Check sheet for the modelled part. Datum: model origin and axes. Units: mm. A direction names the side the tool comes from. Give positions to 0.01 mm unless a question says otherwise; leave off trailing zeros. Order: outer loops, then holes, each group sorted by start corner. A loop starts at its lowest first (then second) coordinate and runs counter-clockwise, first axis right, second up.
```python
from build123d import *

# Parameters (mm, degrees)
SKETCH176_R     = 2.25
PAD098_DEPTH    = 4
SKETCH177_W     = 20.5
SKETCH177_H     = 20.5
POCKET040_DEPTH = 2
CHAMFER002_SIZE = 0.8
FILLET008_R     = 1.5


with BuildPart() as part:
    # Sketch176 → Pad098 (new body)
    with BuildSketch(Plane.YZ):
        with BuildLine():
            ThreePointArc((5.946308, -16.98945), (0, 18), (-5.946308, -16.98945))
            Line((-3.5, -10), (-5.946308, -16.98945))
            ThreePointArc((3.5, -10), (0, -6.5), (-3.5, -10))
            Line((5.946308, -16.98945), (3.5, -10))
        make_face()
        Circle(SKETCH176_R, mode=Mode.SUBTRACT)
        with BuildLine():
            ThreePointArc((-5.663715, 13.673417), (-6.36727, 11.974885), (-4.668738, 11.27133))
            ThreePointArc((4.668738, 11.27133), (0, 12.2), (-4.668738, 11.27133))
            ThreePointArc((4.668738, 11.27133), (6.36727, 11.974885), (5.663715, 13.673417))
            ThreePointArc((5.663715, 13.673417), (0, 14.8), (-5.663715, 13.673417))
        make_face(mode=Mode.SUBTRACT)
    extrude(amount=PAD098_DEPTH)

    # Sketch177 (on Face10 of Pad098) → Pocket040 (cut)
    with BuildSketch(Plane(origin=(0, 0, 0), x_dir=(0, 1, 0), z_dir=(-1, 0, 0))):
        Rectangle(SKETCH177_W, SKETCH177_H)
    extrude(amount=-POCKET040_DEPTH, mode=Mode.SUBTRACT)

    # Chamfer002
    chamfer002_edges = [part.edges().sort_by_distance(p)[0] for p in [
        (0, 6.36727, 11.974885),
        (0, 0, 14.8),
        (0, 0, 12.2),
        (0, -6.36727, 11.974885),
    ]]
    chamfer(chamfer002_edges, length=CHAMFER002_SIZE)

    # Fillet008
    fillet008_edges = [part.edges().sort_by_distance(p)[0] for p in [
        (0, 0, 18),
    ]]
    fillet(fillet008_edges, radius=FILLET008_R)


with BuildPart() as part_1:
    # Body140 placement: moved
    add(part.part.moved(Location((-11, 0, 54))))


solid = part_1.part
```
(1) Material ranges on L1, parallel to Z at x = -8.25, y = 0; L2, parallel to Y at x = -7.6, z = 54; L3, parallel to X at y = -5, z = 61, recorded low to high.
Response values:
L1: z = 47.5 to 51.75, 56.25 to 66.2, 68.8 to 72
L2: y = -18 to -2.25, 2.25 to 18
L3: x = -9 to -7
(2) Release check for a two-part mould opening along Z. For faces 4 (the face through (-10, 10.25, 54)), 5 (the face through (-9.03, 4.74, 40.46)), 6 (the face through (-8.268, 0.707, 71.986)), 7 (the face through (-8.6, 0.1, 68.8)) record: released by +Z, released by -Z, zero draft, split by the parting line, or undercut.
Response values:
face 4: undercut
face 5: released by -Z
face 6: split by the parting line
face 7: undercut
(3) Gauge pin test, flat ends, axial feed: pin 1 Ø2 at (x, z) = (-10, 50) entering from -Y; pin 2 Ø7 at (y, z) = (0, 54) entering from -X; pin 3 Ø0.6 at (x, y) = (-10, 7) entering from +Z. Record the tip position at first contact, or that the pin passes through.
Response values:
pin 1: stops at y = -17.73
pin 2: stops at x = -9
pin 3: stops at z = 70.65
(4) Set-up check for faces 1 (the face through (-9.028, -4.706, 40.554)), 2 (the face through (-8.6, 0.1, 66.2)), 3 (the face through (-10, 0, 64.25)): record each of +Z, -Z, +X, -X, +Y, -Y from which the full face is reachable in a straight line by a thin tool's end or side.
Response values:
face 1: -Z, +X, -X
face 2: +X, -X
face 3: -X
(5) Cross-section at A-A on y = 0. Enter the section's corners in (x, z).
Response values:
outline: (-11, 64.25) - (-9, 64.25) - (-9, 56.25) - (-7, 56.25) - (-7, 66.2) - (-10.2, 66.2) - (-11, 65.4) - close; (-11, 69.6) - (-10.2, 68.8) - (-7, 68.8) - (-7, 72) - (-9.5, 72) arc R1.5 ccw to (-11, 70.5) - close; (-9, 47.5) - (-7, 47.5) - (-7, 51.75) - (-9, 51.75) - close
